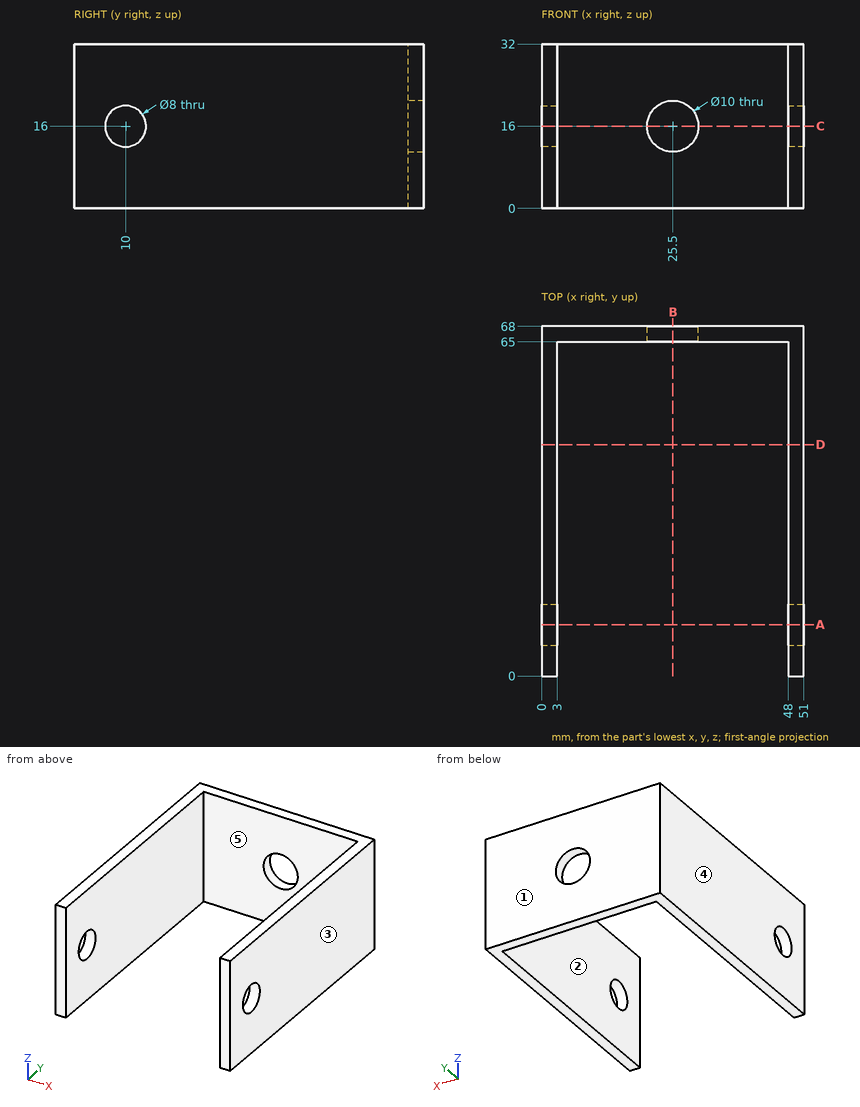
Verification items for this drawing (mm, ordinates from the low corner). A direction names the side the tool comes from. Give positions to 0.01 mm unless a question says otherwise; leave off trailing zeros. Loops run counter-clockwise (first coordinate to the right, second up) from the corner with the lowest first, then second, coordinate; pieces in that order, holes last. Notation, with made-up numbers: M 37,53 L 64,53 A25 cw 64,65 Z; hole C 11,63.5 d5. An arc over 180 degrees is marked long. Write item = value, one per line. Start each with the question number.
1. Draft check along X on the marked faces 3, 4 and 5. Enter one of: +X half, -X half, draft (parallel to the pull), parting line (faces both ways), or undercut.
2. Thickness scan on probe 1 along X at (y, z) = (23, 14.5); probe 2 along X at (y, z) = (66.35, 16); probe 3 along Y at (x, z) = (0.8, 16). Record the ranges inside material, lowest first.
3. Tool access check on the marked faces 1 and 2. Record the directions out of +Z, -Z, +X, -X, +Y, -Y that give a thin tool (end or side, any length) a straight path to the whole face; none if there is none.
4. Section check C-C, the plane z = 16. Enter the section's corners in (x, y), plus the area to 3 significant figures.
5. Section check B-B, the plane x = 25.5. Enter the section's corners in (y, z), plus the area to 3 significant figures.
6. Section check A-A, the plane y = 10. Enter the section's corners in (x, z).
7. Go/stop test with a flat-tipped pin: P1, Ø10, axis at x = 41, z = 18, coming from the -Y side. Record where the tip stops, or that it passes through.
8. Section check D-D, the plane y = 45. Enter the section's corners in (x, z), plus the area to 3 significant figures.
Values follow:
q1.face_3 = +X half
q1.face_4 = -X half
q1.face_5 = undercut
q2.probe_1 = 0 to 3, 48 to 51
q2.probe_2 = 0 to 20.5, 30.5 to 51
q2.probe_3 = 0 to 6, 14 to 68
q3.face_1 = +Z, -Z, +X, -X, +Y
q3.face_2 = +Z, -Z, -Y
q4.outline = M 0,0 L 3,0 L 3,6 L 0,6 Z; M 0,14 L 3,14 L 3,65 L 20.5,65 L 20.5,68 L 0,68 Z; M 30.5,65 L 48,65 L 48,14 L 51,14 L 51,68 L 30.5,68 Z; M 48,0 L 51,0 L 51,6 L 48,6 Z
q4.area = 465 mm^2
q5.outline = M 65,0 L 68,0 L 68,11 L 65,11 Z; M 65,21 L 68,21 L 68,32 L 65,32 Z
q5.area = 66.0 mm^2
q6.outline = M 0,0 L 3,0 L 3,12 L 0,12 Z; M 0,20 L 3,20 L 3,32 L 0,32 Z; M 48,0 L 51,0 L 51,12 L 48,12 Z; M 48,20 L 51,20 L 51,32 L 48,32 Z
q7.P1 = 65
q8.outline = M 0,0 L 3,0 L 3,32 L 0,32 Z; M 48,0 L 51,0 L 51,32 L 48,32 Z
q8.area = 192 mm^2
